```python
from build123d import *

# Parameters (mm, degrees)
SKETCH_1_W          = 12
SKETCH_1_H          = 12
SKETCH_1_W_2        = 10
SKETCH_1_H_2        = 10
EXTRUDE_1_DEPTH     = 200
SKETCH_2_R          = 1
CUT_EXTRUDE_1_DEPTH = 12


with BuildPart() as part:
    # 草图1 → 凸台-拉伸1 (new body)
    with BuildSketch(Plane.XY):
        with Locations((6, 6)):
            Rectangle(SKETCH_1_W, SKETCH_1_H)
        with Locations((6, 6)):
            Rectangle(SKETCH_1_W_2, SKETCH_1_H_2, mode=Mode.SUBTRACT)
    extrude(amount=EXTRUDE_1_DEPTH)

    # 草图2 → 切除-拉伸1 (cut)
    with BuildSketch(Plane.XZ):
        with Locations(Location((6, 190, 0), (0, 0, 270))):
            Circle(SKETCH_2_R)
    extrude(amount=-CUT_EXTRUDE_1_DEPTH, mode=Mode.SUBTRACT)


solid = part.part
```
Can you work these out from the model? Positions are in its coordinate system, mm. A direction names the side the tool comes from. Give positions to 0.01 mm unless a question says otherwise; leave off trailing zeros. Loops run counter-clockwise (first coordinate to the right, second up) from the corner with the lowest first, then second, coordinate; pieces in that order, holes last. Notation, with made-up numbers: M 48.25,64 L 100.25,64 A11 ccw 100.25,85 Z; hole C -38.75,76.25 d3. An arc over 180 degrees is marked long. Use CSV: the item, a comma, the result in double quotes. Start each with the question number.
1. On a 3-axis mill with a long thin cutter (end or side, diameter ignored), from which of +Z, -Z, +X, -X, +Y, -Y can I reach the whole of each face in a straight line? I mean faces 5 (the face through (0, 6, 99)), 6 (the face through (1, 6, 99)). Say none if no direction works.
2. If I drill on L1, parallel to Y at x = 1.5, z = 66.5; L2, parallel to X at y = 0.5, z = 190, over which ranges is the centre line in solid material (lowest first)?
3. Imagine slicing it at B-B, the plane y = 7.5. Write out the boundary of the cut face in (x, z).
4. Imagine slicing it at A-A, the plane z = 47. Write out the boundary of the cut face in (x, y), plus the area to 3 significant figures.
5. If we mould it in two halves opening along Y, with no side actions, what happens to faces 1 (the face through (6, 12, 99)), 2 (the face through (11.2, 6.1, 0)), 3 (the face through (11, 6, 99)), 4 (the face through (6, 11, 99))? For each: released by +Y, released by -Y, zero draft, split by the parting line, or undercut.
Response values:
1,face 5,"+Z, -Z, -X, +Y, -Y"
1,face 6,"+Z, -Z"
2,L1,"0 to 1, 11 to 12"
2,L2,"0 to 5, 7 to 12"
3,outline,"M 0,0 L 1,0 L 1,200 L 0,200 Z; M 11,0 L 12,0 L 12,200 L 11,200 Z"
4,outline,"M 0,0 L 12,0 L 12,12 L 0,12 Z; hole M 1,1 L 11,1 L 11,11 L 1,11 Z"
4,area,"44.0 mm^2"
5,face 1,"released by +Y"
5,face 2,"zero draft"
5,face 3,"undercut"
5,face 4,"undercut"
